Here's how the part is built. I have some questions about the finished solid (model axes, mm). Face numbers are marked on the shaded views. Coordinates: 2 decimals unless noted, no trailing zeros. Write each loop counter-clockwise with the first axis right and the second up, starting at its lowest first coordinate (ties: lowest second). Pieces come first, ordered by that corner, then holes. Notation, with made-up numbers: (51.25, 81) -> (74.25, 81) arc R20 cw to (74.25, 109) -> close; hole circle Ø11 at (-33, 49.25). An arc over 180 degrees is marked (long way). Use a Markdown table: item, result. Add a question column.
```python
from build123d import *

# Parameters (mm, degrees)
SKETCH1_W           = 76
SKETCH1_H           = 55
SKETCH1_W_2         = 64.2
SKETCH1_H_2         = 43.4
BOSS_EXTRUDE1_DEPTH = 4
SKETCH2_W           = 74.2
SKETCH2_H           = 53.4
CUT_EXTRUDE1_DEPTH  = 2
SKETCH3_R           = 1.35
CUT_EXTRUDE2_DEPTH  = 2
CUT_EXTRUDE3_REACH  = 4
SKETCH4_R           = 1.5


with BuildPart() as part:
    # Sketch1 → Boss-Extrude1 (new body)
    with BuildSketch(Plane(origin=(0, 0, 0), x_dir=(1, 0, 0), z_dir=(0, 1, 0))):
        Rectangle(SKETCH1_W, SKETCH1_H)
        Rectangle(SKETCH1_W_2, SKETCH1_H_2, mode=Mode.SUBTRACT)
    extrude(amount=BOSS_EXTRUDE1_DEPTH)

    # Sketch2 → Cut-Extrude1 (cut)
    with BuildSketch(Plane(origin=(0, 4, 0), x_dir=(1, 0, 0), z_dir=(0, 1, 0))):
        Rectangle(SKETCH2_W, SKETCH2_H)
    extrude(amount=-CUT_EXTRUDE1_DEPTH, mode=Mode.SUBTRACT)

    # Sketch3 → Cut-Extrude2 (cut)
    with BuildSketch(Plane(origin=(0, 2, 0), x_dir=(1, 0, 0), z_dir=(0, 1, 0))):
        with Locations((0, 24.2)):
            Circle(SKETCH3_R)
        with Locations((0, -24.2)):
            Circle(SKETCH3_R)
    extrude(amount=-CUT_EXTRUDE2_DEPTH, mode=Mode.SUBTRACT)

    # Sketch4 → Cut-Extrude3 (cut, up to next)
    with BuildSketch(Plane(origin=(0, 2, 0), x_dir=(1, 0, 0), z_dir=(0, 1, 0)), mode=Mode.PRIVATE) as cut_extrude3_sk1:
        with Locations((34.6, 0)):
            Circle(SKETCH4_R)
    cut_extrude3_tool1 = extrude(cut_extrude3_sk1.sketch, amount=-CUT_EXTRUDE3_REACH, mode=Mode.PRIVATE) & part.part
    add(cut_extrude3_tool1.solids().sort_by_distance((34.6, 2, 0))[0], mode=Mode.SUBTRACT)


solid = part.part
```
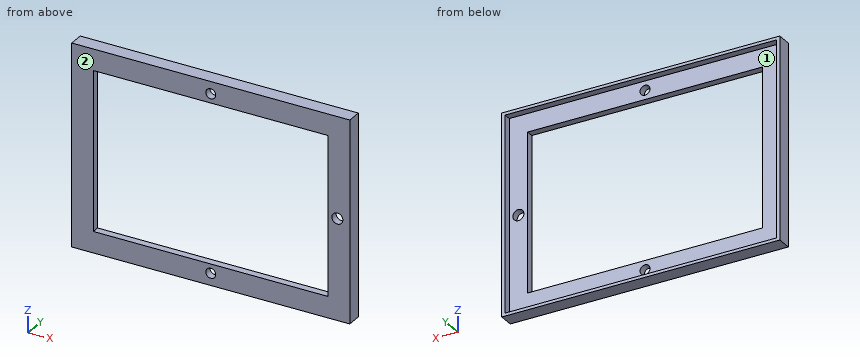
Q1. Will these pins go through, and if not, where does the flat tip stop? pin 1 (5 mm diameter, centred on x = 5.5, z = -20.5, fed in from +Y); pin 2 (1.5 mm diameter, centred on x = 7.5, z = 20, fed in from +Y).
Q2. Please list where these lines run through material, in increasing order: line 1 (X direction, y = 2.1, z = -2); line 2 (X direction, y = 0.55, z = 14); line 3 (X direction, y = 1.2, z = 0).
Q3. Suppose I cut it at D-D, the plane x = 0. Write out the boundary of the cut face in (y, z).
Q4. Thinking about a two-plate mould opening in X: for the marked faces 1 and 2, which applies, released by +X, released by -X, zero draft, split by the parting line, or undercut?
Q5. Suppose I cut it at C-C, the plane z = 0. Write out the boundary of the cut face in (x, y).
Q6. Suppose I cut it at B-B, the plane x = 34.6. Write out the boundary of the cut face in (y, z).
Q7. Suppose I cut it at A-A, the plane z = -6. Write out the boundary of the cut face in (x, y).
Answer key:
| question | item | result |
|---|---|---|
| 1 | pin 1 | stops at y = 2 |
| 1 | pin 2 | passes through |
| 2 | line 1 | x = -38 to -37.1, 37.1 to 38 |
| 2 | line 2 | x = -38 to -32.1, 32.1 to 38 |
| 2 | line 3 | x = -38 to -32.1, 32.1 to 33.1, 36.1 to 38 |
| 3 | outline | (0, -27.5) -> (4, -27.5) -> (4, -26.7) -> (2, -26.7) -> (2, -25.55) -> (0, -25.55) -> close; (0, -22.85) -> (2, -22.85) -> (2, -21.7) -> (0, -21.7) -> close; (0, 21.7) -> (2, 21.7) -> (2, 22.85) -> (0, 22.85) -> close; (0, 25.55) -> (2, 25.55) -> (2, 26.7) -> (4, 26.7) -> (4, 27.5) -> (0, 27.5) -> close |
| 4 | face 1 | undercut |
| 4 | face 2 | zero draft |
| 5 | outline | (-38, 0) -> (-32.1, 0) -> (-32.1, 2) -> (-37.1, 2) -> (-37.1, 4) -> (-38, 4) -> close; (32.1, 0) -> (33.1, 0) -> (33.1, 2) -> (32.1, 2) -> close; (36.1, 0) -> (38, 0) -> (38, 4) -> (37.1, 4) -> (37.1, 2) -> (36.1, 2) -> close |
| 6 | outline | (0, -27.5) -> (4, -27.5) -> (4, -26.7) -> (2, -26.7) -> (2, -1.5) -> (0, -1.5) -> close; (0, 1.5) -> (2, 1.5) -> (2, 26.7) -> (4, 26.7) -> (4, 27.5) -> (0, 27.5) -> close |
| 7 | outline | (-38, 0) -> (-32.1, 0) -> (-32.1, 2) -> (-37.1, 2) -> (-37.1, 4) -> (-38, 4) -> close; (32.1, 0) -> (38, 0) -> (38, 4) -> (37.1, 4) -> (37.1, 2) -> (32.1, 2) -> close |
